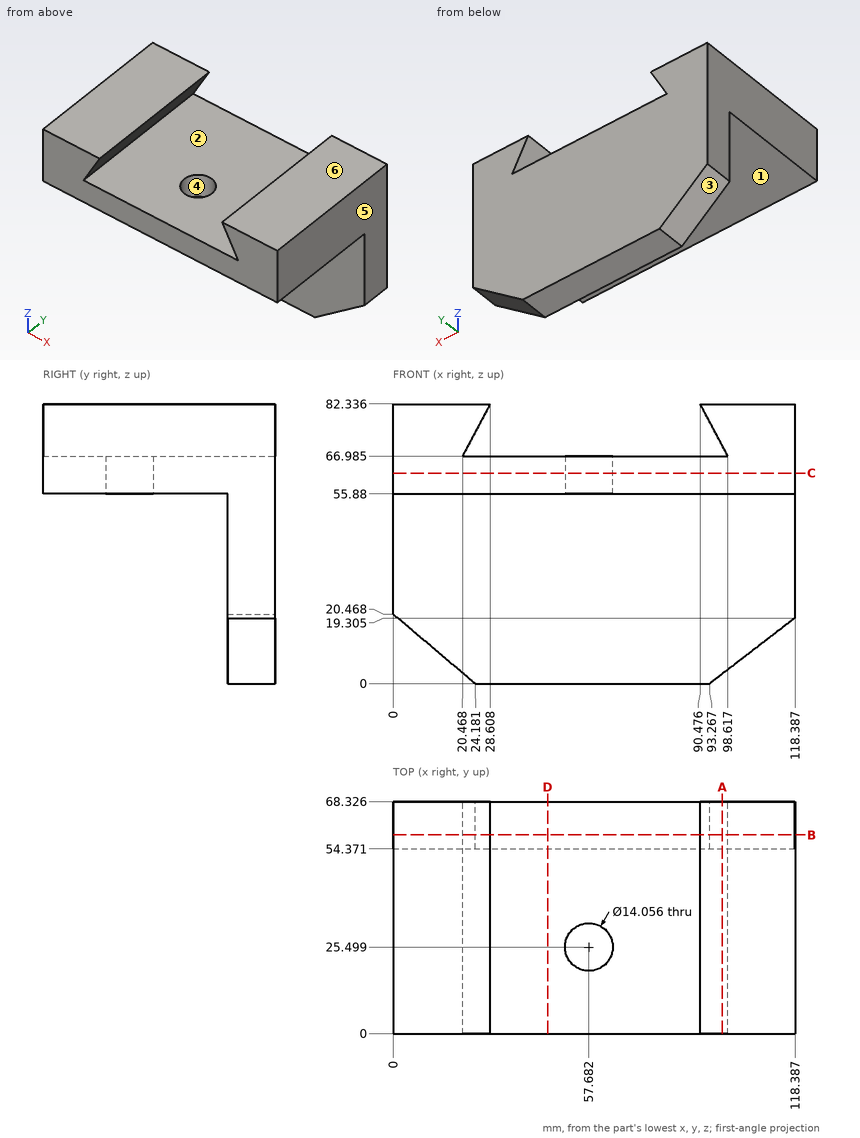
The figure shows three views and two pictorial views of one solid part (mm, origin at its lowest corner). Answer the questions. A direction names the side the tool comes from. Give positions to 0.01 mm unless a question says otherwise; leave off trailing zeros. Write each loop counter-clockwise with the first axis right and the second up, starting at its lowest first coordinate (ties: lowest second). Pieces come first, ordered by that corner, then holes. Notation, with made-up numbers: (73.5, 32) - (130.5, 32) arc R14 ccw to (130.5, 40) - close; hole circle Ø11 at (2, 80.5). An arc over 180 degrees is marked (long way). Use one line per item in the form item = value.
1. Consider L1, parallel to Z at x = 33.5, y = 29 (1 decimal); L2, parallel to Y at x = 24, z = 42; L3, parallel to Y at x = 61, z = 59 (1 decimal). Determine where each line is inside the solid, lowest interval first.
Filled in:
L1 = 55.9 to 67
L2 = 54.37 to 68.33
L3 = 0 to 19.3, 31.7 to 68.3
2. Determine the mould class of the marked faces 4, 5 and 6 for opening direction X: released by +X, released by -X, zero draft, split by the parting line, or undercut.
Filled in:
face_4 = undercut
face_5 = released by +X
face_6 = zero draft
3. Each of these flat-tipped pins is pushed along its axis until it touches: pin 1 Ø5 at (x, y) = (44, 39.5) entering from -Z; pin 2 Ø6 at (x, z) = (15.5, 24.5) entering from -Y. Where does it stop, or does it pass through?
Filled in:
pin_1 = 55.88
pin_2 = 54.37
4. A cutting plane is placed at A-A (x = 97). Write down the section's boundary in (y, z) (1 decimal).
Filled in:
outline = (0, 55.9) - (54.4, 55.9) - (54.4, 2.9) - (68.3, 2.9) - (68.3, 67) - (0, 67) - close; (0, 70) - (68.3, 70) - (68.3, 82.3) - (0, 82.3) - close
5. A cutting plane is placed at D-D (x = 45.5). Write down the section's boundary in (y, z) (1 decimal), and give its area (3 significant figures).
Filled in:
outline = (0, 55.9) - (54.4, 55.9) - (54.4, 0) - (68.3, 0) - (68.3, 67) - (0, 67) - close
area = 1,540 mm^2
6. A cutting plane is placed at C-C (z = 62). Write down the section's boundary in (x, y) (1 decimal), and give its area (3 significant figures).
Filled in:
outline = (0, 0) - (118.4, 0) - (118.4, 68.3) - (0, 68.3) - close; hole circle Ø14.1 at (57.7, 25.5)
area = 7,930 mm^2
7. A cutting plane is placed at B-B (y = 58.5). Write down the section's boundary in (x, z) (1 decimal).
Filled in:
outline = (0, 20.5) - (24.2, 0) - (93.3, 0) - (118.4, 19.3) - (118.4, 82.3) - (90.5, 82.3) - (98.6, 67) - (20.5, 67) - (28.6, 82.3) - (0, 82.3) - close
8. For the marked faces 1, 2 and 3, determine the directions among +Z, -Z, +X, -X, +Y, -Y from which every point of the face is accessible in a straight line to the end or side of a thin tool.
Filled in:
face_1 = -Z, +X, -X, -Y
face_2 = +Y, -Y
face_3 = -Z, -X, +Y, -Y
